Verification items for this drawing (mm, ordinates from the low corner). Give positions to 0.01 mm unless a question says otherwise; leave off trailing zeros. Loops run counter-clockwise (first coordinate to the right, second up) from the corner with the lowest first, then second, coordinate; pieces in that order, holes last. Notation, with made-up numbers: (-1, -1) -> (14, -1) arc R21 cw to (14, 28) -> close; hole circle Ø4 at (32.25, 68). An arc over 180 degrees is marked (long way). Answer in a Markdown table with one row per item. Add a question column.
Q1. Section check C-C on x = 17.75. Enter the section's corners in (y, z), and give its area (3 significant figures).
Q2. Section check B-B on z = 0.65. Give the number of separate pieces and of enclosed holes in the cut face, and give its area (3 significant figures).
Q3. Material ranges on probe 1 along X at (y, z) = (2.4, 1.15); probe 2 along X at (y, z) = (1.9, 2.05); probe 3 along Z at (x, y) = (20.75, 1.9), recorded low to high.
Q4. Section check A-A on x = 1.7. Enter the section's corners in (y, z), and give its area (3 significant figures).
Q5. Gauge pin test, flat end, axial feed: P1, Ø1.5, axis at x = 22, z = 3.5, coming from the -Y side. Record the tip position at first contact, or that the pin passes through.
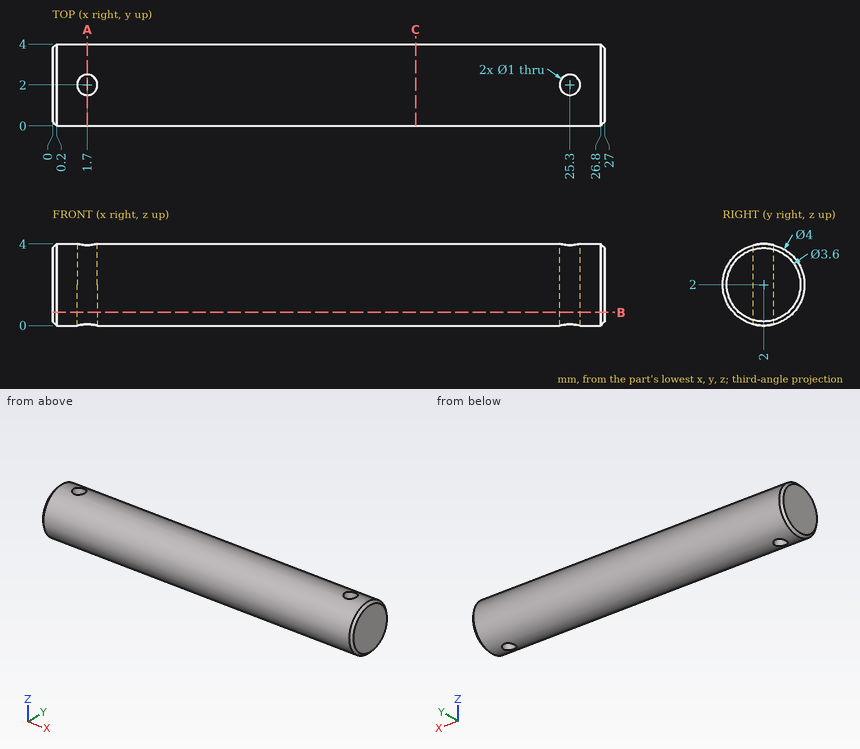
Taken from the geometry:
| question | item | result |
|---|---|---|
| 1 | outline | circle Ø4 at (2, 2) |
| 1 | area | 12.6 mm² |
| 2 | separate pieces | 1 |
| 2 | enclosed holes | 2 |
| 2 | area | 78.0 mm² |
| 3 | probe 1 | x = 0 to 1.4, 2 to 25, 25.6 to 27 |
| 3 | probe 2 | x = 0 to 1.21, 2.19 to 24.81, 25.79 to 27 |
| 3 | probe 3 | z = 0 to 4 |
| 4 | outline | (1.5, 0.06) -> (1.5, 3.94) arc R2 ccw to start; (2.5, 0.06) arc R2 ccw to (2.5, 3.94) -> close |
| 4 | area | 8.61 mm² |
| 5 | P1 | stops at y = 0.15 |
